```python
from build123d import *

# Parameters (mm, degrees)
F0_W          = 125.194638
F0_H          = 65.465718
F1_DEPTH      = 25.4
F2_R          = 8.887572
F2_R_2        = 9.445227
F2_R_3        = 8.938329
F2_R_4        = 11.778548
F3_DEPTH      = 25.4
F4_R          = 10.913086
F5_DEPTH      = 25.4
F5_DEPTH_BACK = 25.4


with BuildPart() as f1:
    # F0 (on Top) → F1 (new body)
    with BuildSketch(Plane.XY):
        Rectangle(F0_W, F0_H)
    extrude(amount=F1_DEPTH)

    # F2 (on face) → F3 (cut)
    with BuildSketch(Plane.XY.offset(25.4)):
        with Locations((34.231201, 15.227929)):
            Circle(F2_R)
        with Locations((-40.088922, 16.693249)):
            Circle(F2_R_2)
        with Locations((32.400653, -16.642913)):
            Circle(F2_R_3)
        with Locations((-41.187249, -15.543923)):
            Circle(F2_R_4)
    extrude(amount=-F3_DEPTH, mode=Mode.SUBTRACT)

    # F4 (on face) → F5 (cut, two sides)
    with BuildSketch(Plane.XY.offset(25.4)) as f5_sk:
        with Locations((0, -7.362174)):
            Circle(F4_R)
    extrude(amount=-F5_DEPTH, mode=Mode.SUBTRACT)
    extrude(f5_sk.sketch, amount=-F5_DEPTH_BACK, mode=Mode.SUBTRACT)


solid = f1.part
```
Input: part model. Units: mm. Frame: model coordinates. Give positions to 0.01 mm unless a question says otherwise; leave off trailing zeros. Order: outer loops, then holes, each group sorted by start corner. A loop starts at its lowest first (then second) coordinate and runs counter-clockwise, first axis right, second up.
1. Section C-C on y = -23.5. Return the cut outline in (x, z).
Derived:
outline: (-62.6, 0) - (-49.87, 0) - (-49.87, 25.4) - (-62.6, 25.4) - close; (-32.5, 0) - (26.67, 0) - (26.67, 25.4) - (-32.5, 25.4) - close; (38.13, 0) - (62.6, 0) - (62.6, 25.4) - (38.13, 25.4) - close
2. Section A-A on x = 0. Return the cut outline in (y, z).
Derived:
outline: (-32.73, 0) - (-18.28, 0) - (-18.28, 25.4) - (-32.73, 25.4) - close; (3.55, 0) - (32.73, 0) - (32.73, 25.4) - (3.55, 25.4) - close
3. Section D-D on z = 11.25. Return the cut outline in (x, y).
Derived:
outline: (-62.6, -32.73) - (62.6, -32.73) - (62.6, 32.73) - (-62.6, 32.73) - close; hole circle Ø23.56 at (-41.19, -15.54); hole circle Ø18.89 at (-40.09, 16.69); hole circle Ø21.83 at (0, -7.36); hole circle Ø17.88 at (32.4, -16.64); hole circle Ø17.78 at (34.23, 15.23)
4. Mould query, pull axis Y, two halves, no side actions, for faces 1 (the flat face through (-62.597, 0, 13)), 2 (the flat face through (-1, -32.733, 13)), 3 (the cylindrical face through (23.47, -16.25, 12.88)). Classes: released by +Y, released by -Y, zero draft, split by the parting line, or undercut.
Derived:
face 1: zero draft
face 2: released by -Y
face 3: undercut
5. Pin query (flat end, axial travel): pin 1 (12 mm diameter, centred on x = 41.5, y = -9.5, fed in from -Z); pin 2 (10.5 mm diameter, centred on x = 32.4, y = -16.64, fed in from -Z). Return the tip coordinate at first contact, or that it passes through.
Derived:
pin 1: stops at z = 0
pin 2: passes through
6. Material intervals for L1, parallel to X at y = -9, z = 22.25; L2, parallel to Y at x = 29.5, z = 15.75; L3, parallel to X at y = 16, z = 20, sorted ascending.
Derived:
L1: x = -62.6 to -50.98, -31.39 to -10.79, 10.79 to 27.77, 37.04 to 62.6
L2: y = -32.73 to -25.1, -8.19 to 7.7, 22.75 to 32.73
L3: x = -62.6 to -49.51, -30.67 to 25.38, 43.09 to 62.6
7. Section B-B on y = -0.5. Return the cut outline in (x, z), and give its area (3 significant figures).
Derived:
outline: (-62.6, 0) - (-8.49, 0) - (-8.49, 25.4) - (-62.6, 25.4) - close; (8.49, 0) - (62.6, 0) - (62.6, 25.4) - (8.49, 25.4) - close
area: 2,750 mm2
